```python
from build123d import *

# Parameters (mm, degrees)
BOSS_EXTRUDE1_DEPTH = 50.8
SKETCH2_W           = 12.7
SKETCH2_H           = 6.35
BOSS_EXTRUDE2_DEPTH = 6.35
SKETCH3_R           = 1.499997
CUT_EXTRUDE1_DEPTH  = 71.299547696
FILLET1_R           = 2.54
FILLET2_R           = 25.4


with BuildPart() as part:
    # Sketch1 → Boss-Extrude1 (new body)
    with BuildSketch(Plane(origin=(0, 0, 0), x_dir=(0, 0, -1), z_dir=(1, 0, 0))):
        Polygon((0, 0), (-42.8625, 0), (-42.8625, 4.7625), (-4.7625, 4.7625), (-4.7625, 30.1625), (0, 30.1625), align=None)
    extrude(amount=BOSS_EXTRUDE1_DEPTH)

    # Sketch2 → Boss-Extrude2 (add)
    with BuildSketch(Plane(origin=(0, 4.7625, 0), x_dir=(1, 0, 0), z_dir=(0, 1, 0))):
        with Locations((25.4, -20.6375)):
            Rectangle(SKETCH2_W, SKETCH2_H)
    extrude(amount=BOSS_EXTRUDE2_DEPTH)

    # Sketch3 → Cut-Extrude1 (cut, through all)
    with BuildSketch(Plane.XY.offset(4.7625)):
        with Locations((25.4, 23.8125)):
            Circle(SKETCH3_R)
    extrude(amount=-CUT_EXTRUDE1_DEPTH, mode=Mode.SUBTRACT)

    # Fillet1
    fillet1_edges = [part.edges().sort_by_distance(p)[0] for p in [
        (19.05, 11.1125, 20.6375),
        (25.4, 11.1125, 23.8125),
        (31.75, 11.1125, 20.6375),
        (25.4, 11.1125, 17.4625),
    ]]
    fillet(fillet1_edges, radius=FILLET1_R)

    # Fillet2
    fillet2_edges = [part.edges().sort_by_distance(p)[0] for p in [
        (50.8, 30.1625, 2.38125),
        (0, 30.1625, 2.38125),
    ]]
    fillet(fillet2_edges, radius=FILLET2_R - 0.0001)  # a hair under: the kernel refuses the full size


solid = part.part
```
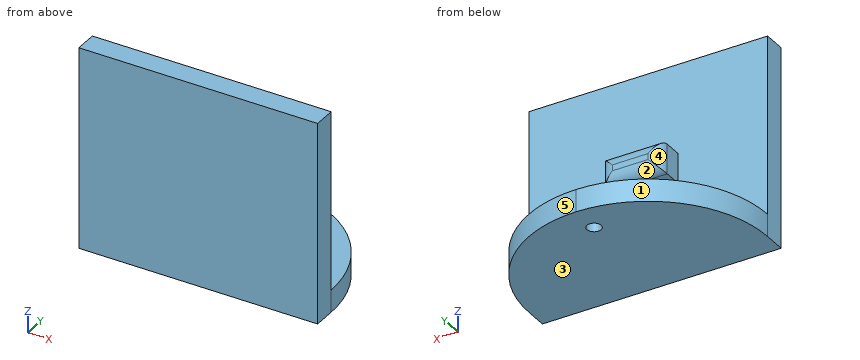
Could you check a few things on this model? Use its own coordinates, in mm. Face numbers are marked on the shaded views. A direction names the side the tool comes from. Coordinates: 2 decimals unless noted, no trailing zeros. Write each loop counter-clockwise with the first axis right and the second up, starting at its lowest first coordinate (ties: lowest second). Pieces come first, ordered by that corner, then holes. Notation, with made-up numbers: (35.25, 40.5) -> (50.25, 40.5) arc R32 cw to (50.25, 71.5) -> close; hole circle Ø9 at (0, -3.75). An arc over 180 degrees is marked (long way). One line per question, with ' | ' between items. Start each with the question number.
1. If we section it at A-A (y = 6): Please give me the cut outline in (x, z), and give its area (3 significant figures).
2. If we section it at B-B (x = 30.5): Please give me the cut outline in (y, z), and give its area (3 significant figures).
3. If we section it at D-D (y = 10): Please give me the cut outline in (x, z).
4. For the marked faces 4 and 5, which set-ups out of +Z, -Z, +X, -X, +Y, -Y let a thin tool reach every point of the face, with its end or its side?
5. Will these pins go through, and if not, where does the flat tip stop? P1, Ø12.5, axis at x = 33, y = 22.5, coming from the +Z side; P2, Ø1.9, axis at x = 26.5, y = 6.5, coming from the +Z side; P3, Ø6, axis at x = 41, z = 21.5, coming from the +Y side; P4, Ø3, axis at y = 6, z = 21.5, coming from the -X side.
6. If we section it at C-C (z = 29.5): Please give me the cut outline in (x, y).
7. Please list where these lines run through material, in increasing order: line 1 along Z through (x, y) = (7.5, 8); line 2 along Y through (x, z) = (27, 20.5); line 3 along Z through (x, y) = (29, 7.5).
8. Thinking about a two-plate mould opening in Z: for the marked faces 1, 2 and 3, which applies, pulls with the +Z half, pulls with the -Z half, needs draft (parallel to the pull), parting line crosses it, or undercut?
Return value:
1) outline: (0.03, 0) -> (50.77, 0) -> (50.77, 4.76) -> (0.03, 4.76) -> close; (19.05, 17.46) -> (31.75, 17.46) -> (31.75, 23.81) -> (19.05, 23.81) -> close | area: 322 mm²
2) outline: (0, 0) -> (29.65, 0) -> (29.65, 4.76) -> (4.76, 4.76) -> (4.76, 17.46) -> (8.57, 17.46) arc R2.54 ccw to (10.76, 18.71) -> (10.76, 22.56) arc R2.54 ccw to (8.57, 23.81) -> (4.76, 23.81) -> (4.76, 42.86) -> (0, 42.86) -> close | area: 359 mm²
3) outline: (0.55, 0) -> (50.25, 0) -> (50.25, 4.76) -> (0.55, 4.76) -> close; (19.49, 17.9) -> (31.31, 17.9) -> (31.31, 23.37) -> (19.49, 23.37) -> close
4) face 4: +Z, -X, +Y | face 5: +Z, -Z, +X, +Y
5) P1: stops at z = 4.76 | P2: stops at z = 23.81 | P3: stops at y = 4.76 | P4: stops at x = 0
6) outline: (0, 0) -> (50.8, 0) -> (50.8, 4.76) -> (0, 4.76) -> close
7) line 1: z = 0 to 4.76 | line 2: y = 0 to 11.11 | line 3: z = 0 to 4.76, 17.46 to 23.81
8) face 1: needs draft | face 2: undercut | face 3: pulls with the -Z half
